Check sheet for the drawn part. Datum: minimum x, y, z corner. Units: mm. Round coordinates to 2 decimals unless told otherwise and drop trailing zeros. Write each loop counter-clockwise with the first axis right and the second up, starting at its lowest first coordinate (ties: lowest second). Pieces come first, ordered by that corner, then holes.
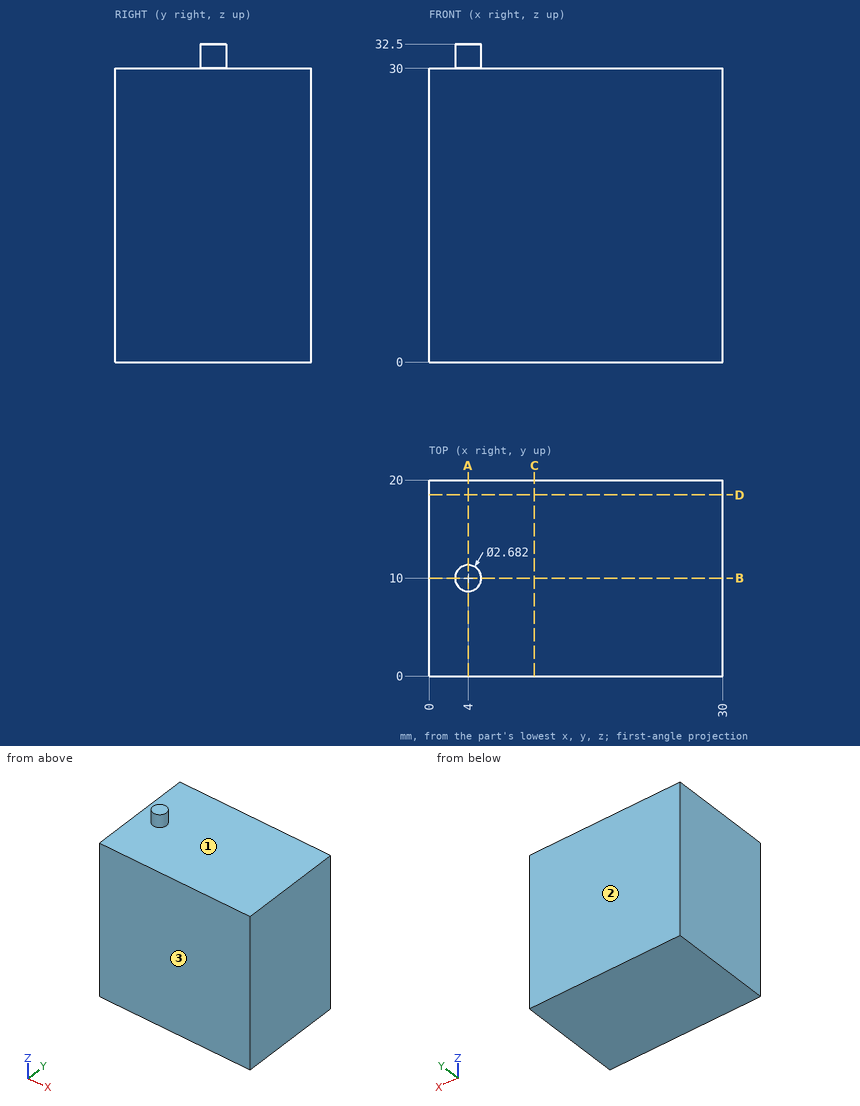
Q1. Release check for a two-part mould opening along Y. For the marked faces 1, 2 and 3 record: released by +Y, released by -Y, zero draft, split by the parting line, or undercut.
Recorded:
face 1: zero draft
face 2: released by +Y
face 3: released by -Y
Q2. Material ranges on line 1 along Z through (x, y) = (11.5, 16.5); line 2 along Y through (x, z) = (4.75, 30.5), recorded low to high.
Recorded:
line 1: z = 0 to 30
line 2: y = 8.89 to 11.11
Q3. Sectioned sample at A-A (x = 4). Enter the section's corners in (y, z), plus the area to 3 significant figures.
Recorded:
outline: (0, 0) - (20, 0) - (20, 30) - (11.34, 30) - (11.34, 32.5) - (8.66, 32.5) - (8.66, 30) - (0, 30) - close
area: 607 mm2
Q4. Sectioned sample at D-D (y = 18.5). Enter the section's corners in (x, z).
Recorded:
outline: (0, 0) - (30, 0) - (30, 30) - (0, 30) - close
Q5. Depth check by flat-ended pin: P1, Ø12, axis at x = 19.5, y = 11.5, coming from the +Z side. Enter the tip coordinate at first touch or a pass-through.
Recorded:
P1: stops at z = 30
Q6. Sectioned sample at C-C (x = 10.75). Enter the section's corners in (y, z), plus the area to 3 significant figures.
Recorded:
outline: (0, 0) - (20, 0) - (20, 30) - (0, 30) - close
area: 600 mm2
Q7. Sectioned sample at B-B (y = 10). Enter the section's corners in (x, z), plus the area to 3 significant figures.
Recorded:
outline: (0, 0) - (30, 0) - (30, 30) - (5.34, 30) - (5.34, 32.5) - (2.66, 32.5) - (2.66, 30) - (0, 30) - close
area: 907 mm2
